Geometry: final body of the model. Coordinates: model frame, mm. A direction names the side the tool comes from. Give positions to 0.01 mm unless a question says otherwise; leave off trailing zeros. Loops run counter-clockwise (first coordinate to the right, second up) from the corner with the lowest first, then second, coordinate; pieces in that order, holes last. Notation, with made-up numbers: (32, 29.5) -> (40, 29.5) arc R28 cw to (40, 47.5) -> close; hole circle Ø2 at (5, -16.75). An arc over 180 degrees is marked (long way). Answer in a Markdown table with one row per item. Add a question column.
1) Section query D-D (z = -54). Return the cut outline in (x, y), plus the area to 3 significant figures.
2) Section query A-A (y = 32). Return the cut outline in (x, z).
3) Line query: line 1 (X direction, y = 40.5, z = 2); line 2 (Z direction, x = 26.5, y = 47); line 3 (Y direction, x = -46, z = -53). Output: solid intervals per line, ascending. Write a range as from..to.
4) Section query B-B (z = 38.5). Return the cut outline in (x, y), plus the area to 3 significant figures.
5) Access query for faces 1 (the flat face through (91.998, -2, 15)), 2 (the flat face through (100, 35.5, 10)), 3 (the flat face through (8, 36, 81.556)). Directions: +Z, -Z, +X, -X, +Y, -Y. A direction counts if a zero-diameter tool reaches every point of the face in a straight line with its end or side. Return the directions, or none.
6) First-contact query: P1, Ø2.5, axis at y = 55, z = 10.5, coming from the +X side. Flat tip, straight axial feed; report the tip coordinate or a pass-through.
7) Section query C-C (x = -3.5). Return the cut outline in (y, z).
8) Draft query along Y for faces 4 (the cylindrical face through (73.472, 56.352, -62.584)), 5 (the flat face through (6, -2, -48.694)). Return one class per face: +Y half, -Y half, draft (parallel to the pull), parting line (faces both ways), or undercut.
```python
from build123d import *

# Parameters (mm, degrees)
SKETCH1_W           = 189.996176074
SKETCH1_H           = 150.112754898
BOSS_EXTRUDE1_DEPTH = 60
SKETCH2_W           = 189.996176074
SKETCH2_H           = 150.112754898
BOSS_EXTRUDE2_DEPTH = 4
SKETCH3_W           = 169.42
SKETCH3_H           = 125.25
CUT_EXTRUDE1_DEPTH  = 4
SKETCH4_W           = 15
SKETCH4_H           = 15
CUT_EXTRUDE2_DEPTH  = 222
SKETCH6_W           = 15
SKETCH6_H           = 15
CUT_EXTRUDE3_DEPTH  = 50
SKETCH7_R           = 2
CUT_EXTRUDE4_DEPTH  = 220
SKETCH8_R           = 2
CUT_EXTRUDE5_DEPTH  = 220


with BuildPart() as part:
    # Sketch1 → Boss-Extrude1 (new body)
    with BuildSketch(Plane(origin=(0, 0, 0), x_dir=(1, 0, 0), z_dir=(0, 1, 0))):
        with Locations((7, -10.5)):
            Rectangle(SKETCH1_W, SKETCH1_H)
        Polygon((97.998088037, 60.556377449), (97.998088037, -81.556377449), (-83.998088037, -81.556377449), (-83.998088037, 60.556377449), (16.315151501, 60.556377449), align=None, mode=Mode.SUBTRACT)
    extrude(amount=BOSS_EXTRUDE1_DEPTH)

    # Sketch2 → Boss-Extrude2 (add)
    with BuildSketch(Plane.XZ):
        with Locations((7, 10.5)):
            Rectangle(SKETCH2_W, SKETCH2_H)
    extrude(amount=BOSS_EXTRUDE2_DEPTH)

    # Sketch3 → Cut-Extrude1 (cut)
    with BuildSketch(Plane(origin=(0, 0, 0), x_dir=(1, 0, 0), z_dir=(0, 1, 0))):
        with Locations((7.288088037, -13.931377449)):
            Rectangle(SKETCH3_W, SKETCH3_H)
    extrude(amount=-CUT_EXTRUDE1_DEPTH, mode=Mode.SUBTRACT)

    # Sketch4 → Cut-Extrude2 (cut)
    with BuildSketch(Plane.ZY.offset(87.998088037)):
        with Locations((10.498622551, 28)):
            Rectangle(SKETCH4_W, SKETCH4_H)
    extrude(amount=-CUT_EXTRUDE2_DEPTH, mode=Mode.SUBTRACT)

    # Sketch6 → Cut-Extrude3 (cut)
    with BuildSketch(Plane.XY.offset(85.556377449)):
        with Locations((7.001911963, 28)):
            Rectangle(SKETCH6_W, SKETCH6_H)
    extrude(amount=-CUT_EXTRUDE3_DEPTH, mode=Mode.SUBTRACT)

    # Sketch7 → Cut-Extrude4 (cut)
    with BuildSketch(Plane(origin=(101.998088037, 0, 0), x_dir=(0, 0, -1), z_dir=(1, 0, 0))):
        with Locations((-65.556377449, 55)):
            Circle(SKETCH7_R)
        with Locations((-10.501377449, 55)):
            Circle(SKETCH7_R)
        with Locations((44.556377449, 55)):
            Circle(SKETCH7_R)
    extrude(amount=-CUT_EXTRUDE4_DEPTH, mode=Mode.SUBTRACT)

    # Sketch8 → Cut-Extrude5 (cut)
    with BuildSketch(Plane(origin=(0, 0, -64.556377449), x_dir=(-1, 0, 0), z_dir=(0, 0, -1))):
        with Locations((-71.998088037, 55)):
            Circle(SKETCH8_R)
        with Locations((-6.998088037, 55)):
            Circle(SKETCH8_R)
        with Locations((57.998088037, 55)):
            Circle(SKETCH8_R)
    extrude(amount=-CUT_EXTRUDE5_DEPTH, mode=Mode.SUBTRACT)


solid = part.part
```
Evaluation:
| question | item | result |
|---|---|---|
| 1 | outline | (-88, -4) -> (102, -4) -> (102, 60) -> (98, 60) -> (98, 0) -> (-84, 0) -> (-84, 60) -> (-88, 60) -> close |
| 1 | area | 1,240 mm² |
| 2 | outline | (-88, -64.56) -> (102, -64.56) -> (102, 3) -> (98, 3) -> (98, -60.56) -> (-84, -60.56) -> (-84, 3) -> (-88, 3) -> close; (-88, 18) -> (-84, 18) -> (-84, 81.56) -> (-0.5, 81.56) -> (-0.5, 85.56) -> (-88, 85.56) -> close; (14.5, 81.56) -> (98, 81.56) -> (98, 18) -> (102, 18) -> (102, 85.56) -> (14.5, 85.56) -> close |
| 3 | line 1 | -88..-84, 98..102 |
| 3 | line 2 | -64.56..-60.56, 81.56..85.56 |
| 3 | line 3 | -4..0 |
| 4 | outline | (-88, -4) -> (-77.42, -4) -> (-77.42, 0) -> (-84, 0) -> (-84, 60) -> (-88, 60) -> close; (92, -4) -> (102, -4) -> (102, 60) -> (98, 60) -> (98, 0) -> (92, 0) -> close |
| 4 | area | 562 mm² |
| 5 | face 1 | +Y, -Y |
| 5 | face 2 | +X, -X |
| 5 | face 3 | +Y |
| 6 | P1 | through |
| 7 | outline | (-4, -64.56) -> (60, -64.56) -> (60, -60.56) -> (0, -60.56) -> (0, -48.69) -> (-4, -48.69) -> close; (-4, 76.56) -> (0, 76.56) -> (0, 81.56) -> (60, 81.56) -> (60, 85.56) -> (-4, 85.56) -> close |
| 8 | face 4 | undercut |
| 8 | face 5 | draft |
